Input: dimensioned drawing with shaded views. Units: mm. Origin: part minimum x, y, z. A direction names the side the tool comes from. Give positions to 0.01 mm unless a question says otherwise; leave off trailing zeros. Loops run counter-clockwise (first coordinate to the right, second up) from the corner with the lowest first, then second, coordinate; pieces in that order, holes last.
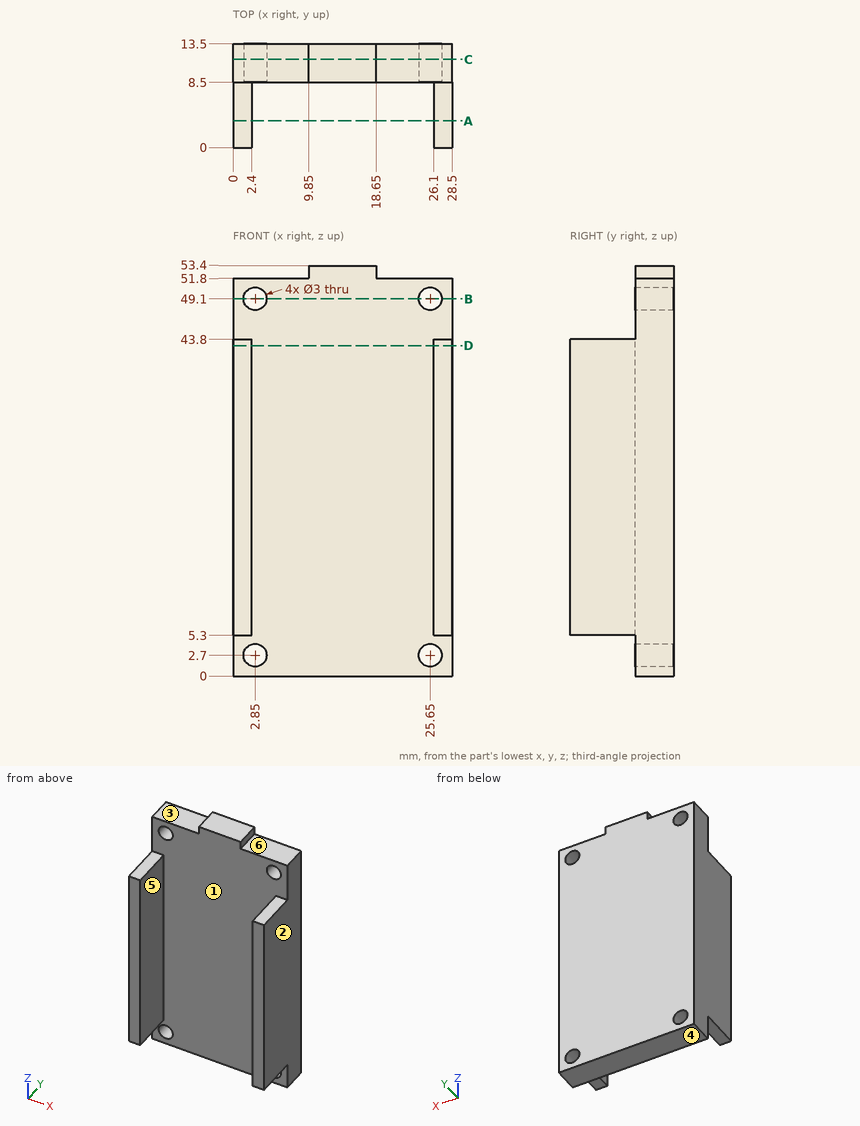
(1) Reachability of the marked faces 4, 5 and 6 from +Z, -Z, +X, -X, +Y, -Y: full face, straight path, thin tool, end or side. Return the list, or none.
A:
face 4: -Z, +X, -X, +Y, -Y
face 5: +Z, -Z, -Y
face 6: +Z, +X, +Y, -Y
(2) Ray query, line 1 along X through (y, z) = (11.75, 49.1); line 2 along X through (y, z) = (5, 16.5); line 3 along Y through (x, z) = (15.25, 7.5). Return the intervals inside material, ascending.
A:
line 1: x = 0 to 1.35, 4.35 to 24.15, 27.15 to 28.5
line 2: x = 0 to 2.4, 26.1 to 28.5
line 3: y = 8.5 to 13.5
(3) Section D-D, the plane z = 43. Return the cut outline in (x, y).
A:
outline: (0, 0) - (2.4, 0) - (2.4, 8.5) - (26.1, 8.5) - (26.1, 0) - (28.5, 0) - (28.5, 13.5) - (0, 13.5) - close
(4) Section A-A, the plane y = 3.5. Return the cut outline in (x, z).
A:
outline: (0, 5.3) - (2.4, 5.3) - (2.4, 43.8) - (0, 43.8) - close; (26.1, 5.3) - (28.5, 5.3) - (28.5, 43.8) - (26.1, 43.8) - close
(5) Mould query, pull axis X, two halves, no side actions, for the marked faces 1, 2 and 3. Classes: pulls with the +X half, pulls with the -X half, needs draft (parallel to the pull), parting line crosses it, or undercut.
A:
face 1: undercut
face 2: pulls with the +X half
face 3: needs draft
(6) Section B-B, the plane z = 49.1. Return the cut outline in (x, y).
A:
outline: (0, 8.5) - (1.35, 8.5) - (1.35, 13.5) - (0, 13.5) - close; (4.35, 8.5) - (24.15, 8.5) - (24.15, 13.5) - (4.35, 13.5) - close; (27.15, 8.5) - (28.5, 8.5) - (28.5, 13.5) - (27.15, 13.5) - close
(7) First-contact query: pin 1 (0.7 mm diameter, centred on x = 27.5, y = 4.5, fed in from +Z); pin 2 (1.5 mm diameter, centred on x = 25.5, y = 12, fed in from +Z); pin 3 (1.3 mm diameter, centred on y = 11, z = 52.5, fed in from -X). Flat tips, straight axial feed; report the tip coordinate or a pass-through.
A:
pin 1: stops at z = 43.8
pin 2: stops at z = 51.8
pin 3: stops at x = 9.85
(8) Section C-C, the plane y = 11.5. Return the cut outline in (x, z), then the cut area to 3 significant figures.
A:
outline: (0, 0) - (28.5, 0) - (28.5, 51.8) - (18.65, 51.8) - (18.65, 53.4) - (9.85, 53.4) - (9.85, 51.8) - (0, 51.8) - close; hole circle Ø3 at (2.85, 2.7); hole circle Ø3 at (2.85, 49.1); hole circle Ø3 at (25.65, 2.7); hole circle Ø3 at (25.65, 49.1)
area: 1,460 mm2
